Verification items for the finished model (mm, model axes). Face numbers are marked on the shaded views. A direction names the side the tool comes from. Round coordinates to 2 decimals unless told otherwise and drop trailing zeros. Write each loop counter-clockwise with the first axis right and the second up, starting at its lowest first coordinate (ties: lowest second). Pieces come first, ordered by that corner, then holes. Notation, with made-up numbers: (-18, 67) - (4, 67) arc R31 cw to (4, 94) - close; hole circle Ø4 at (64.25, -34). An arc over 180 degrees is marked (long way). Answer as a JSON object with one key per item and string values.
```python
from build123d import *

# Parameters (mm, degrees)
BASE_DEPTH           = 10
ESQUISSE5_R          = 2.5
VIDE_ACCES_VIS_DEPTH = 30.434846638
BOSS_START           = -5
ESQUISSE6_R          = 8.5
ESQUISSE6_R_2        = 2.5
BOSS_VIS_DEPTH       = 5
ESQUISSE7_R          = 6.25
VIDE_ECROU_DEPTH     = 2.5


with BuildPart() as part:
    # Esquisse2 → BASE (new body)
    with BuildSketch(Plane(origin=(0, 0, 0), x_dir=(0, 0, -1), z_dir=(1, 0, 0))):
        with BuildLine():
            Line((-26.180339887, 10), (-16.717843024, 10))
            Line((-16.717843024, 10), (-14.361406616, 10))
            Line((-14.361406616, 10), (-11.180339887, 10))
            ThreePointArc((-11.180339887, 10), (0, 15), (11.180339887, 10))
            Line((11.180339887, 10), (14.361406616, 10))
            Line((14.361406616, 10), (20.155156542, 10))
            Line((20.155156542, 10), (21.180339887, 10))
            Line((21.180339887, 10), (26.180339887, 10))
            Line((26.180339887, 10), (26.180339887, 15))
            Line((26.180339887, 15), (11.66190379, 15))
            ThreePointArc((11.66190379, 15), (0, 19), (-11.66190379, 15))
            Line((-11.66190379, 15), (-26.180339887, 15))
            Line((-26.180339887, 15), (-26.180339887, 10))
        make_face()
    extrude(amount=BASE_DEPTH)

    # Esquisse5 → VIDE ACCES VIS (cut, through all)
    with BuildSketch(Plane.XZ.offset(-10)):
        with Locations(Location((5, 21.180339887, 0), (0, 0, 270))):
            Circle(ESQUISSE5_R)
        with Locations(Location((5, -21.180339887, 0), (0, 0, 270))):
            Circle(ESQUISSE5_R)
    extrude(amount=-VIDE_ACCES_VIS_DEPTH, mode=Mode.SUBTRACT)

    # Esquisse6 → BOSS VIS (add)
    # profile 1 of 2: a face of its own
    with BuildSketch(Plane(origin=(0, 15, 0), x_dir=(1, 0, 0), z_dir=(0, 1, 0)).offset(BOSS_START)):
        with Locations((5, -21.180339887)):
            Circle(ESQUISSE6_R)
        with Locations(Location((5, -21.180339887, 0), (0, 0, 90))):
            Circle(ESQUISSE6_R_2, mode=Mode.SUBTRACT)
    # profile 2 of 2: a face of its own
    with BuildSketch(Plane(origin=(0, 15, 0), x_dir=(1, 0, 0), z_dir=(0, 1, 0)).offset(BOSS_START)):
        with Locations((5, 21.180339887)):
            Circle(ESQUISSE6_R)
        with Locations(Location((5, 21.180339887, 0), (0, 0, 90))):
            Circle(ESQUISSE6_R_2, mode=Mode.SUBTRACT)
    extrude(amount=BOSS_VIS_DEPTH)

    # Esquisse7 → VIDE ECROU (cut)
    with BuildSketch(Plane(origin=(0, 15, 0), x_dir=(1, 0, 0), z_dir=(0, 1, 0))):
        with Locations(Location((5, 21.180339887, 0), (0, 0, 270))):
            Circle(ESQUISSE7_R)
        with Locations(Location((5, -21.180339887, 0), (0, 0, 270))):
            Circle(ESQUISSE7_R)
    extrude(amount=-VIDE_ECROU_DEPTH, mode=Mode.SUBTRACT)


solid = part.part
```
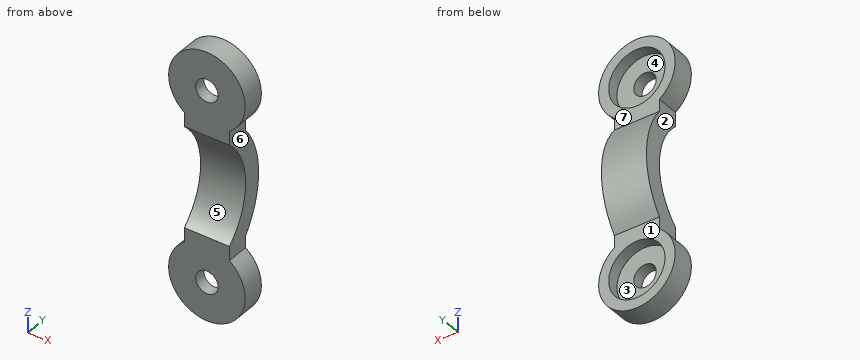
1. Cross-section at A-A (x = 5). Record the boundary of the cut face in (y, z).
Completed:
{"outline": "(10, -29.68) - (15, -29.68) - (15, -27.43) - (12.5, -27.43) - (12.5, -23.68) - (10, -23.68) - close; (10, -18.68) - (12.5, -18.68) - (12.5, -14.93) - (15, -14.93) - (15, -11.66) arc R19 ccw to (15, 11.66) - (15, 14.93) - (12.5, 14.93) - (12.5, 18.68) - (10, 18.68) - (10, 11.18) arc R15 cw to (10, -11.18) - close; (10, 23.68) - (12.5, 23.68) - (12.5, 27.43) - (15, 27.43) - (15, 29.68) - (10, 29.68) - close"}
2. Cross-section at B-B (y = 11). Record the boundary of the cut face in (x, z).
Completed:
{"outline": "(0, -14.31) arc R8.5 ccw (long way) to (10, -14.31) - (10, -10.2) - (0, -10.2) - close; (0, 10.2) - (10, 10.2) - (10, 14.31) arc R8.5 ccw (long way) to (0, 14.31) - close; hole circle Ø5 at (5, -21.18); hole circle Ø5 at (5, 21.18)"}
3. Cross-section at C-C (y = 13.5). Record the boundary of the cut face in (x, z), plus the area to 3 significant figures.
Completed:
{"outline": "(0, -14.31) arc R8.5 ccw (long way) to (10, -14.31) - (10, -6.54) - (0, -6.54) - close; (0, 6.54) - (10, 6.54) - (10, 14.31) arc R8.5 ccw (long way) to (0, 14.31) - close; hole circle Ø12.5 at (5, -21.18); hole circle Ø12.5 at (5, 21.18)", "area": "342 mm^2"}
4. Go/stop test with flat-tipped pins: pin 1 (2 mm diameter, centred on x = 0, y = 17.5, fed in from -Z); pin 2 (5 mm diameter, centred on x = 8, z = 23.5, fed in from +Y); pin 3 (3 mm diameter, centred on x = 8, y = 13.5, fed in from +Z). Record where each tip stops, or that it passes through.
Completed:
{"pin 1": "stops at z = -9.42", "pin 2": "stops at y = 15", "pin 3": "stops at z = 29.55"}
5. Cross-section at D-D (z = -17). Record the boundary of the cut face in (x, y), plus the area to 3 significant figures.
Completed:
{"outline": "(-2.4, 10) - (12.4, 10) - (12.4, 15) - (9.65, 15) - (9.65, 12.5) - (0.35, 12.5) - (0.35, 15) - (-2.4, 15) - close", "area": "50.8 mm^2"}
6. Access from +Z, -Z, +X, -X, +Y, -Y to the whole of each face (thin tool, end or side, straight path). Record for the marked faces 5, 6 and 7.
Completed:
{"face 5": "+X, -X, -Y", "face 6": "+X, +Y, -Y", "face 7": "+Z, +X, -X, +Y"}
7. Mould release check, pull along X, two halves, no side actions. Record for the marked faces 1, 2, 3 and 4: released by +X, released by -X, zero draft, split by the parting line, or undercut.
Completed:
{"face 1": "zero draft", "face 2": "released by -X", "face 3": "undercut", "face 4": "undercut"}
8. Material ranges on probe 1 along Z at (x, y) = (8.25, 12.75); probe 2 along Z at (x, y) = (5.25, 11.75); probe 3 along Y at (x, z) = (3.5, -13.5), recorded low to high. Write a range as from..to.
Completed:
{"probe 1": "z = -29.03..-26.52, -15.84..-7.9, 7.9..15.84, 26.52..29.03", "probe 2": "z = -29.68..-23.67, -18.69..-9.32, 9.32..18.69, 23.67..29.68", "probe 3": "y = 10..15"}
